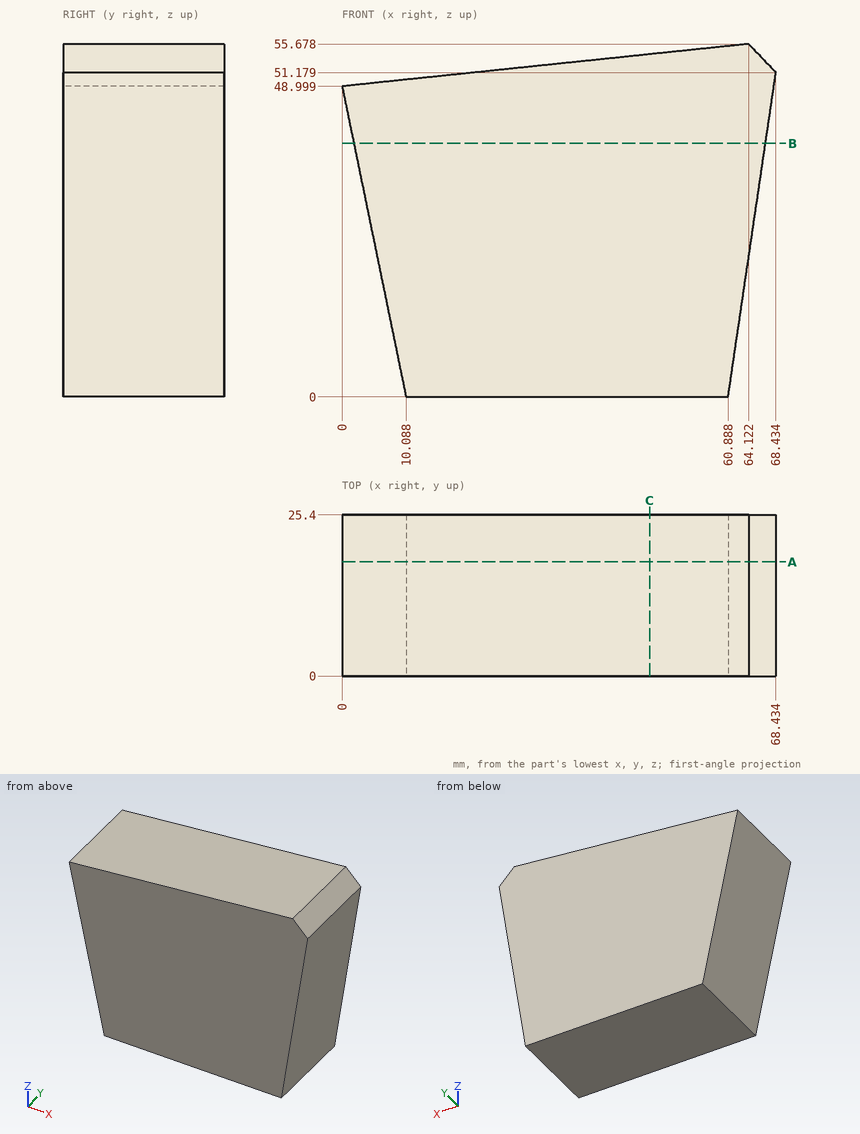
The drawing under review shows one solid part. Ordinate dimensions are in mm from its lowest x, y, z. Give positions to 0.01 mm unless a question says otherwise; leave off trailing zeros. Write each loop counter-clockwise with the first axis right and the second up, starting at its lowest first coordinate (ties: lowest second). Pieces come first, ordered by that corner, then holes. Notation, with made-up numbers: M -4,-0.75 L 46,-0.75 A29 ccw 46,26.25 Z; hole C 5.25,2.5 d11. An arc over 180 degrees is marked long. Write each question's results on one line, items separated by ' | '. Start each with the question number.
1. We need section A-A (y = 18). Write out the cut boundary in (x, z).
2. We need section B-B (z = 40). Write out the cut boundary in (x, y).
3. We need section C-C (x = 48.5). Write out the cut boundary in (y, z), and give its area (3 significant figures).
4. Insertion check: pin 1 Ø4 at (x, y) = (26.5, 17.5) entering from -Z; pin 2 Ø6 at (y, z) = (13.5, 12) entering from +X; pin 3 Ø1.5 at (y, z) = (5, 11) entering from -X; pin 4 Ø12 at (x, y) = (10.5, 8.5) entering from +Z. Each pin has a flat end and moves straight along its axis. Give the tip position at first contact, or say it passes through.
5. For probe 1 along Z at (x, y) = (30.5, 2.25); probe 2 along X at (y, z) = (2, 5) (1 decimal); probe 3 along X at (y, z) = (14.75, 32), list the stretches that pass through material, from the lowest coordinate up. Write a range as [from, to].
Results found:
1) outline: M 0,49 L 10.09,0 L 60.89,0 L 68.43,51.18 L 64.12,55.68 Z
2) outline: M 1.85,0 L 66.79,0 L 66.79,25.4 L 1.85,25.4 Z
3) outline: M 0,0 L 25.4,0 L 25.4,54.05 L 0,54.05 Z | area: 1,370 mm^2
4) pin 1: stops at z = 0 | pin 2: stops at x = 63.1 | pin 3: stops at x = 7.67 | pin 4: stops at z = 50.72
5) probe 1: z = [0, 52.18] | probe 2: x = [9.1, 61.6] | probe 3: x = [3.5, 65.61]
